Design review of the part built by this model. Coordinates are the model's own, in mm. A direction names the side the tool comes from. Coordinates: 2 decimals unless noted, no trailing zeros. Write each loop counter-clockwise with the first axis right and the second up, starting at its lowest first coordinate (ties: lowest second). Pieces come first, ordered by that corner, then holes. Notation, with made-up numbers: (19, 21) - (23, 21) arc R34 ccw to (23, 54) - close; hole circle Ø9 at (81.25, 31). An arc over 180 degrees is marked (long way). Answer as CSV lines item,"result". Start each with the question number.
Q1. We need section D-D (x = 12.5). Write out the cut boundary in (y, z).
Q2. We need section C-C (y = 2). Write out the cut boundary in (x, z).
Q3. Machinability: for faces 4 (the face through (-15.53, 1.97, 3.48)), 5 (the face through (5.18, 4.88, -1.08)), 6 (the face through (-17.5, -2, -4)), which of the approach directions +Z, -Z, +X, -X, +Y, -Y give a long, thin tool a straight path to every point of the face, cutting with its end or side? Answer none if there is none.
Q4. We need section B-B (x = -11.5). Write out the cut boundary in (y, z), plus the area to 3 significant figures.
Q5. Clearance check with flat-ended pins moving along their axes: pin 1 (2 mm diameter, centred on x = 12.5, z = -4, fed in from -Y); pin 2 (2 mm diameter, centred on x = -5, z = 0.5, fed in from +Y); pin 3 (3 mm diameter, centred on x = -15, z = -1, fed in from +Y); pin 4 (1 mm diameter, centred on x = 0.5, z = -1, fed in from -Y). State where each tip first meets the part, or that it passes through.
Q6. Mouldability with a two-part tool opening along Z and no side actions: class faces 1 (the face through (17.5, 0, 0)), 2 (the face through (-12.43, 7.81, -1.73)), 3 (the face through (-16, 4, 0)) as pulls with the +Z half, pulls with the -Z half, needs draft (parallel to the pull), parting line crosses it, or undercut.
Q7. For line 1 along X through (y, z) = (0.5, -2.5); line 2 along X through (y, z) = (6.5, 0.25); line 3 along Y through (x, z) = (-12.5, 6.25), list the stretches that pass through material, from the lowest coordinate up. Write a range as [from, to].
Q8. We need section A-A (z = 0). Write out the cut boundary in (x, y).
Solid Edge part; units mm, degrees
sketch "Sketch1" plane through (10.8674, 0, 10.8674) normal (0, -1, 0) x (1, 0, 0)
  line L0 (-28.3674, -10.8674) -> (-28.3674, -2.8674)
  line L1 (-28.3674, -2.8674) -> (-18.3674, -2.8674)
  line L2 (-18.3674, -2.8674) -> (-18.3674, -5.8674)
  line L3 (-18.3674, -5.8674) -> (6.6326, -5.8674)
  line L4 (6.6326, -5.8674) -> (6.6326, -10.8674)
revolve "RevolvedProtrusion1" add sketch "Sketch1" angle 360 about axis through (16.5, 0, 0) along (-1, 0, 0)
sketch "Sketch2" plane through (-17.5, 0, 0) normal (-1, 0, 0) x (0, 0, -1)
  line L0 (4.6188, 0) -> (2.3094, 4)
  line L1 (2.3094, 4) -> (-2.3094, 4)
  line L2 (-2.3094, 4) -> (-4.6188, 0)
  line L3 (-4.6188, 0) -> (-2.3094, -4)
  line L4 (-2.3094, -4) -> (2.3094, -4)
  line L5 (2.3094, -4) -> (4.6188, 0)
extrude "Cutout1" cut sketch "Sketch2" against normal blind 4
cosmetic_thread "Thread1"
properties material "Steel"
Results list:
1,outline,"circle Ø10 at (0, 0)"
2,outline,"(-17.5, -7.75) - (-7.5, -7.75) - (-7.5, -4.58) - (17.5, -4.58) - (17.5, 4.58) - (-7.5, 4.58) - (-7.5, 7.75) - (-17.5, 7.75) - (-17.5, 3.46) - (-13.5, 3.46) - (-13.5, -3.46) - (-17.5, -3.46) - close"
3,face 4,"-X"
3,face 5,"+X"
3,face 6,"+Z, -Z, -X, +Y, -Y"
4,outline,"circle Ø16 at (0, 0)"
4,area,"201 mm2"
5,pin 1,"stops at y = -4"
5,pin 2,"stops at y = 5"
5,pin 3,"stops at y = 8"
5,pin 4,"stops at y = -4.97"
6,face 1,"needs draft"
6,face 2,"parting line crosses it"
6,face 3,"undercut"
7,line 1,"x = [-13.5, 17.5]"
7,line 2,"x = [-17.5, -7.5]"
7,line 3,"y = [-4.99, 4.99]"
8,outline,"(-17.5, -8) - (-7.5, -8) - (-7.5, -5) - (17.5, -5) - (17.5, 5) - (-7.5, 5) - (-7.5, 8) - (-17.5, 8) - (-17.5, 4) - (-13.5, 4) - (-13.5, -4) - (-17.5, -4) - close"
